Autodesk Inventor part; units mm, degrees
ref_plane "Work Plane1" through (0, 0, 6.35) normal (0, 0, 1) x (1, 0, 0)
ref_plane "YZ Plane" through (0, 0, 0) normal (1, 0, 0) x (0, 1, 0)
ref_plane "XZ Plane" through (0, 0, 0) normal (0, 1, 0) x (-1, 0, 0)
sketch "Sketch1" plane through (0, 0, 0) normal (0, 0, 1) x (1, 0, 0)
  circle A0 centre (0, 0) radius 3
  line L0 (-1.6129, 1.6129) -> (1.6129, 1.6129)
  line L1 (1.6129, 1.6129) -> (1.6129, -1.6129)
  line L2 (1.6129, -1.6129) -> (-1.6129, -1.6129)
  line L3 (-1.6129, -1.6129) -> (-1.6129, 1.6129)
  dimension "d0" = 6
  dimension "d1" = 3.2258
  dimension "d2" = 3.2258
  dimension "d3" = 1.6129
  dimension "d4" = 1.6129
extrude "Extrusion1" add sketch "Sketch1" along normal blind 12.7
ref_plane "Work Plane1" through (0, 0, 6.35) normal (0, 0, 1) x (1, 0, 0)
sketch "Sketch2" plane through (0, 0, 6.35) normal (0, 0, 1) x (1, 0, 0)
  circle A0 centre (0, 0) radius 3
extrude "Extrusion2" add sketch "Sketch2" along normal mid plane 3.175
chamfer "Chamfer1" distance 0.254 angle 45 2 edges at (-3, 0, 0) (-3, 0, 12.7)
properties part number "Vex Shaft Coupler" material "Steel"
For this review, take the finished solid that the model builds, in its own axes (mm). A direction names the side the tool comes from. Round coordinates to 2 decimals unless told otherwise and drop trailing zeros. Order: outer loops, then holes, each group sorted by start corner. A loop starts at its lowest first (then second) coordinate and runs counter-clockwise, first axis right, second up. Notation, with made-up numbers: M 3,61.25 L 51,61.25 A19 ccw 51,79.25 Z; hole C 85,84.5 d6. An arc over 180 degrees is marked long. Use a Markdown table: item, result. Add a question column.
Item 1: To check wall thickness, follow line 1 along Y through (x, z) = (1.2, 8.25); line 2 along Z through (x, y) = (-0.4, 1.3); line 3 along X through (y, z) = (-0.9, 9.5). State the ranges of each line that lie inside material, in increasing order.
Item 2: Add section D-D, the plane z = 7.5. Give the boundary of the cut face in (x, y).
Item 3: Insertion check: pin 1 (1.5 mm diameter, centred on x = 2, z = 11, fed in from +Y); pin 2 (3 mm diameter, centred on x = 2, z = 5.5, fed in from -Y); pin 3 (1 mm diameter, centred on x = 0, y = 0.5, fed in from -Z). Each pin has a flat end and moves straight along its axis. Give the tip position at first contact, or say it passes through.
Item 4: Mouldability with a two-part tool opening along X and no side actions: class faces 1 (the flat face through (0, -2, 12.7)), 2 (the flat face through (-1.613, 0, 2)), 3 (the cylindrical face through (-3, 0, 6)) as released by +X, released by -X, zero draft, split by the parting line, or undercut.
Item 5: Add section B-B, the plane z = 10. Give the boundary of the cut face in (x, y), then the cut area to 3 significant figures.
Item 6: Tool access review of faces 4 (the flat face through (0, -2, 0)), 5 (the flat face through (0, -1.613, 2)), 6 (the flat face through (0, -1.613, 10)): name each direction out of +Z, -Z, +X, -X, +Y, -Y from which nothing blocks a thin tool from reaching the whole face with its end or side.
Geometry results:
| question | item | result |
|---|---|---|
| 1 | line 1 | y = -2.75 to -1.61, 1.61 to 2.75 |
| 1 | line 2 | z = 4.76 to 7.94 |
| 1 | line 3 | x = -2.86 to -1.61, 1.61 to 2.86 |
| 2 | outline | C 0,0 d6 |
| 3 | pin 1 | stops at y = 2.73 |
| 3 | pin 2 | stops at y = -2.96 |
| 3 | pin 3 | stops at z = 4.76 |
| 4 | face 1 | zero draft |
| 4 | face 2 | undercut |
| 4 | face 3 | split by the parting line |
| 5 | outline | C 0,0 d6; hole M -1.61,-1.61 L 1.61,-1.61 L 1.61,1.61 L -1.61,1.61 Z |
| 5 | area | 17.9 mm² |
| 6 | face 4 | -Z, +X, -X, +Y, -Y |
| 6 | face 5 | -Z |
| 6 | face 6 | +Z |
